Work out the finished part from the listing and answer in its coordinate system (mm). Face numbers are marked on the shaded views. A direction names the side the tool comes from. Coordinates: 2 decimals unless noted, no trailing zeros. Order: outer loops, then holes, each group sorted by start corner. A loop starts at its lowest first (then second) coordinate and runs counter-clockwise, first axis right, second up. Notation, with made-up numbers: (-13.75, 51.25) -> (45.25, 51.25) arc R33 cw to (45.25, 82.25) -> close; hole circle Ø2 at (41.5, 8.5). An arc over 180 degrees is marked (long way). Answer as CSV lines item,"result". Start each with the question number.
Item 1: Section D-D (x = -557) is taken. Write down the section's boundary in (y, z), then the cut area to 3 significant figures.
Item 2: Section C-C (z = -269) is taken. Write down the section's boundary in (x, y).
Item 3: Section A-A (y = -41) is taken. Write down the section's boundary in (x, z).
Item 4: Which of the six approach directions +Z, -Z, +X, -X, +Y, -Y give full straight-line access (tool end or side, diameter ignored) to the marked faces 1 and 2?
Item 5: Section B-B (x = -691) is taken. Write down the section's boundary in (y, z).
Item 6: Straight lines are drawn through the part: L1, parallel to X at y = -130, z = -568; L2, parallel to Y at x = -212, z = -81; L3, parallel to Z at x = -650.5, y = -134. For each, find the intervals that lie inside material, in ascending order.
Item 7: Each of these flat-tipped pins is pushed along its axis until it touches: pin 1 Ø5 at (x, y) = (-496, -30.5) entering from -Z; pin 2 Ø5 at (y, z) = (-54.5, -573) entering from +X; pin 3 Ø12 at (x, z) = (-206.5, -132.5) entering from +Y. Where does it stop, or does it pass through?
```python
from build123d import *

# Parameters (mm, degrees)
F1_DEPTH = 100
F3_DEPTH = 10
F5_D     = 14
F5_DEPTH = 150


with BuildPart() as f1:
    # F0 (on Front) → F1 (new body)
    with BuildSketch(Plane.XZ):
        Polygon((-70.776085, -70.907202), (-70.776085, 70.645211), (-706.58298, -566.339556), (-565.292317, -566.339556), align=None)
    extrude(amount=F1_DEPTH)

    # F2 (on face) → F3 (join)
    with BuildSketch(Plane(origin=(0, 0, -566.339556), x_dir=(1, 0, 0), z_dir=(0, 0, -1))):
        Polygon((-565.292317, -50), (-565.292317, 100), (-565.292317, 150), (-765.292317, 150), (-765.292317, -50), align=None)
    extrude(amount=F3_DEPTH)

    # F5
    with Locations(Plane(origin=(0, 0, -576.339556), x_dir=(1, 0, 0), z_dir=(0, 0, -1))):
        with Locations((-735.292317, 130), (-595.292317, 130), (-595.292317, -30), (-735.292317, -30)):
            Hole(F5_D / 2, depth=F5_DEPTH)


solid = f1.part
```
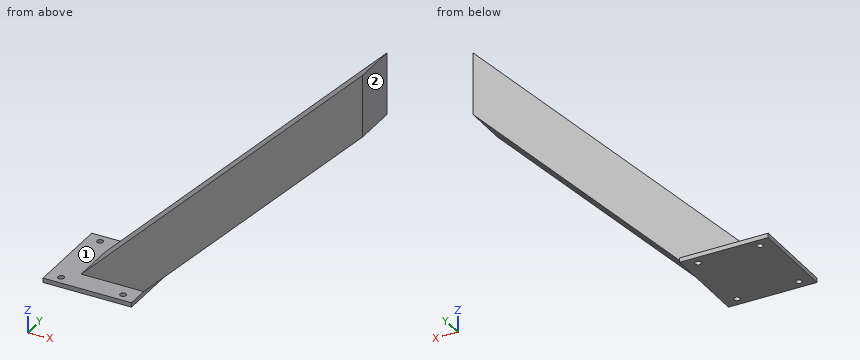
Checked values:
1,outline,"(-100, -558.03) -> (0, -558.03) -> (0, -416.48) -> (-100, -416.48) -> close"
1,area,"14,200 mm^2"
2,outline,"(-409.79, -100) -> (-268.5, -100) -> (-268.5, 0) -> (-409.79, 0) -> close"
3,outline,"(-765.29, -576.34) -> (-565.29, -576.34) -> (-565.29, -566.34) -> (-70.78, -70.91) -> (-70.78, 70.65) -> (-706.58, -566.34) -> (-765.29, -566.34) -> close"
4,face 1,"+Z, -X"
4,face 2,"+Z, -Z, +X, +Y, -Y"
5,outline,"(-150, -576.34) -> (50, -576.34) -> (50, -566.34) -> (0, -566.34) -> (0, -550.73) -> (-100, -550.73) -> (-100, -566.34) -> (-150, -566.34) -> close"
6,L1,"x = -765.29 to -742.29, -728.29 to -602.29, -588.29 to -565.29"
6,L2,"y = -100 to 0"
6,L3,"z = -576.34 to -566.34"
7,pin 1,"stops at z = -499.42"
7,pin 2,"stops at x = -565.29"
7,pin 3,"stops at y = 0"
